Autodesk Inventor part; units mm, degrees
ref_plane "YZ Plane" through (0, 0, 0) normal (1, 0, 0) x (0, 1, 0)
ref_plane "XZ Plane" through (0, 0, 0) normal (0, 1, 0) x (-1, 0, 0)
ref_plane "XY Plane" through (0, 0, 0) normal (0, 0, 1) x (1, 0, 0)
sketch "Sketch1" plane through (0, 0, 0) normal (0, 0, 1) x (1, 0, 0)
  line L0 (0, 49) -> (0, -49) construction
  line L1 (-74, 0) -> (94, 0) construction
  line L2 (-50, -35) -> (70, -35)
  line L3 (70, -35) -> (70, 35)
  line L4 (70, 35) -> (-50, 35)
  line L5 (-50, 35) -> (-50, -35)
  point P0 (0, 0)
  dimension "d4" = 70
  dimension "d49" = 120
  dimension "d50" = 50
  dimension "d51" = 35
extrude "Extrusion3" add sketch "Sketch1" along normal blind 15
sketch "Sketch2" plane through (0, 0, 15) normal (0, 0, 1) x (1, 0, 0)
  point P0 (0, 0)
  point P1 (0, -25)
  point P2 (0, 25)
  dimension "d15" = 25
  dimension "d16" = 25
hole "Hole1" at (0, -25, 15) at (0, 25, 15) direction (0, 0, -1) diameter 6.6 end through all counterbore diameter 11 counterbore depth 6.6
sketch "Sketch3" plane through (0, 0, 15) normal (0, 0, 1) x (1, 0, 0)
  point P0 (0, 0)
  point P1 (-37.5, -12.5)
  point P2 (-37.5, 12.5)
  dimension "d24" = 25
  dimension "d25" = 12.5
  dimension "d26" = 37.5
hole "Hole2" at (-37.5, -12.5, 15) at (-37.5, 12.5, 15) direction (0, 0, -1) diameter 4.917 end through all
sketch "Sketch4" plane through (0, 0, 0) normal (0, 0, -1) x (-1, 0, 0)
  point P0 (0, 0)
  point P1 (10, -10)
  point P2 (-10, 10)
  dimension "d34" = 10
  dimension "d35" = 10
  dimension "d36" = 10
  dimension "d37" = 10
hole "Hole3" at (-10, -10, 0) at (10, 10, 0) direction (0, 0, 1) diameter 5.5 end through all counterbore diameter 10 counterbore depth 5.5
sketch "Sketch5" plane through (0, 0, 15) normal (0, 0, 1) x (1, 0, 0)
  point P0 (0, 0)
  point P1 (10, -10)
  point P2 (-10, 10)
  dimension "d45" = 10
  dimension "d46" = 10
  dimension "d47" = 10
  dimension "d48" = 10
hole "Hole4" at (10, -10, 15) at (-10, 10, 15) direction (0, 0, -1) diameter 4 depth 10 tip angle 118
sketch "Sketch6" plane through (70, -35, 0) normal (1, 0, 0) x (0, 0, -1)
  line L0 (0, 0) -> (-15, 0)
  line L1 (0, 0) -> (0, 70)
  point P0 (0, 35)
  point P1 (-7.5, 15)
  point P2 (-7.5, 55)
  point P3 (-7.5, 0)
  point P4 (0, 35)
  point P5 (0, 35)
  dimension "d59" = 20
  dimension "d60" = 20
hole "Hole5" at (70, -20, 7.5) at (70, 20, 7.5) direction (-1, 0, 0) diameter 4.134 depth 15 tip angle 118
properties part number "23-0064 Base plate" material "ALMg4,5Mn-5083-(D54S)"
Read the model definition and answer for the solid it produces. Units are mm, in the model's axes. A direction names the side the tool comes from. Give positions to 0.01 mm unless a question says otherwise; leave off trailing zeros. Write each loop counter-clockwise with the first axis right and the second up, starting at its lowest first coordinate (ties: lowest second). Pieces come first, ordered by that corner, then holes. Notation, with made-up numbers: M 68.5,-10 L 125.5,-10 A9 cw 125.5,7 Z; hole C 58,3.25 d4. An arc over 180 degrees is marked long. Put each result on its own line as item: value. Start each with the question number.
1. Each of these flat-tipped pins is pushed along its axis until it touches: pin 1 Ø3 at (x, y) = (-9.5, -8.5) entering from -Z; pin 2 Ø10.5 at (x, y) = (0, -25) entering from +Z; pin 3 Ø1.5 at (y, z) = (-21, 7.5) entering from +X. Where does it stop, or does it pass through?
2. The part is cut by section B-B, the plane z = 13.75. Give the number of separate pieces and of enclosed holes in the cut face, and give its area (3 significant figures).
3. The part is cut by section C-C, the plane y = -25. Give the vertices of the cut face in (x, z).
4. For a pull along Y with two mould halves and no side action, classify faces 1 (the conical face through (53.974, 19.682, 7.334)), 2 (the flat face through (9, 0, 0)) as released by +Y, released by -Y, zero draft, split by the parting line, or undercut.
5. The part is cut by section A-A, the plane x = -37.5. Give the vertices of the cut face in (y, z), and give its area (3 significant figures).
6. Consider line 1 along Y through (x, z) = (-37.5, 9.25); line 2 along Y through (x, z) = (0, 12.25); line 3 along X through (y, z) = (-10, 8.5). Determine where each line is inside the solid, lowest interval first.
7. Which of the six approach directions +Z, -Z, +X, -X, +Y, -Y give full straight-line access (tool end or side, diameter ignored) to faces 3 (the cylindrical face through (62.4, -22.05, 7.77)), 4 (the cylindrical face through (8.5, 14.77, 2.79)), 5 (the cylindrical face through (8, -10, 10))?
Final values:
1. pin 1: stops at z = 5.5
1. pin 2: stops at z = 8.4
1. pin 3: stops at x = 54.81
2. separate pieces: 1
2. enclosed holes: 8
2. area: 8,100 mm²
3. outline: M -50,0 L -3.3,0 L -3.3,8.4 L -5.5,8.4 L -5.5,15 L -50,15 Z; M 3.3,0 L 70,0 L 70,15 L 5.5,15 L 5.5,8.4 L 3.3,8.4 Z
4. face 1: undercut
4. face 2: zero draft
5. outline: M -35,0 L -14.96,0 L -14.96,15 L -35,15 Z; M -10.04,0 L 10.04,0 L 10.04,15 L -10.04,15 Z; M 14.96,0 L 35,0 L 35,15 L 14.96,15 Z
5. area: 902 mm²
6. line 1: y = -35 to -14.96, -10.04 to 10.04, 14.96 to 35
6. line 2: y = -35 to -30.5, -19.5 to 19.5, 30.5 to 35
6. line 3: x = -50 to -12.75, -7.25 to 8, 12 to 70
7. face 3: +X
7. face 4: -Z
7. face 5: +Z
